from build123d import *

# Parameters (mm, degrees)
EXTRUDE_1_DEPTH     = 6
EXTRUDE_2_DEPTH     = 20
SKETCH_3_W          = 25
SKETCH_3_H          = 50
EXTRUDE_3_DEPTH     = 3
EXTRUDE_4_DEPTH     = 6
SKETCH_5_R          = 1
CUT_EXTRUDE_1_DEPTH = 74.184697854


with BuildPart() as part:
    # 草图1 → 凸台-拉伸1 (new body)
    with BuildSketch(Plane(origin=(0, 0, 0), x_dir=(1, 0, 0), z_dir=(0, 1, 0))):
        with BuildLine():
            Line((5, 0), (5, -13))
            Line((5, -13), (-15, -13))
            Line((-15, -13), (-15, -63))
            Line((-15, -63), (10, -63))
            Line((10, -63), (10, -66))
            Line((10, -66), (-18, -66))
            Line((-18, -66), (-18, -10))
            Line((-18, -10), (-5, -10))
            Line((-5, -10), (-5, 0))
            ThreePointArc((-5, 0), (0, 5), (5, 0))
        make_face()
    extrude(amount=-EXTRUDE_1_DEPTH)

    # 草图2 → 凸台-拉伸2 (add, symmetric)
    with BuildSketch(Plane(origin=(0, 0, 0), x_dir=(1, 0, 0), z_dir=(0, 1, 0))):
        Polygon((-15, -13), (5, -13), (5, -10), (-18, -10), (-18, -66), (10, -66), (10, -63), (-15, -63), align=None)
    extrude(amount=EXTRUDE_2_DEPTH, both=True)

    # 草图3 → 凸台-拉伸3 (add)
    with BuildSketch(Plane.XZ.offset(20)):
        with Locations((-2.5, 38)):
            Rectangle(SKETCH_3_W, SKETCH_3_H)
    extrude(amount=-EXTRUDE_3_DEPTH)

    # 草图4 → 凸台-拉伸4 (add)
    with BuildSketch(Plane.XZ.offset(6)):
        with BuildLine():
            ThreePointArc((0.860680542, 8.706562468), (0.72579344, 9.898750182), (0.24342364, 10.997306258))
            ThreePointArc((0.24342364, 10.997306258), (-0.01511058, 10.999989621), (-0.273636452, 10.996595977))
            ThreePointArc((-0.273636452, 10.996595977), (-0.752986286, 9.896718796), (-0.884597491, 8.704164996))
            ThreePointArc((-0.884597491, 8.704164996), (-1.380514283, 8.639397046), (-1.871919927, 8.546397884))
            ThreePointArc((-1.871919927, 8.546397884), (-2.368611449, 9.638553371), (-3.166844887, 10.53428182))
            ThreePointArc((-3.166844887, 10.53428182), (-3.413554747, 10.456942383), (-3.658378768, 10.373825947))
            ThreePointArc((-3.658378768, 10.373825947), (-3.77438681, 9.179653342), (-3.531037114, 8.00479718))
            ThreePointArc((-3.531037114, 8.00479718), (-3.982667613, 7.789952483), (-4.421283831, 7.549652329))
            ThreePointArc((-4.421283831, 7.549652329), (-5.231160146, 8.434867801), (-6.267120572, 9.040088481))
            ThreePointArc((-6.267120572, 9.040088481), (-6.477856391, 8.890296766), (-6.685013481, 8.735593555))
            ThreePointArc((-6.685013481, 8.735593555), (-6.426324056, 7.564019461), (-5.831834222, 6.521864044))
            ThreePointArc((-5.831834222, 6.521864044), (-6.194969688, 6.177973095), (-6.537861669, 5.813894202))
            ThreePointArc((-6.537861669, 5.813894202), (-7.58164644, 6.405518601), (-8.753926829, 6.660988295))
            ThreePointArc((-8.753926829, 6.660988295), (-8.908060318, 6.453406959), (-9.057272497, 6.242260401))
            ThreePointArc((-9.057272497, 6.242260401), (-8.449207929, 5.207966653), (-7.561770763, 4.400525414))
            ThreePointArc((-7.561770763, 4.400525414), (-7.800864967, 3.961250657), (-8.014468055, 3.509031603))
            ThreePointArc((-8.014468055, 3.509031603), (-9.189988356, 3.74915261), (-10.383837737, 3.629864165))
            ThreePointArc((-10.383837737, 3.629864165), (-10.466281235, 3.384812715), (-10.542942575, 3.137891306))
            ThreePointArc((-10.542942575, 3.137891306), (-9.64502446, 2.342121783), (-8.551508496, 1.848432697))
            ThreePointArc((-8.551508496, 1.848432697), (-8.643157232, 1.356773404), (-8.706562468, 0.860680542))
            ThreePointArc((-8.706562468, 0.860680542), (-9.898750182, 0.72579344), (-10.997306258, 0.24342364))
            ThreePointArc((-10.997306258, 0.24342364), (-10.999989621, -0.01511058), (-10.996595977, -0.273636452))
            ThreePointArc((-10.996595977, -0.273636452), (-9.896718796, -0.752986286), (-8.704164996, -0.884597491))
            ThreePointArc((-8.704164996, -0.884597491), (-8.639397046, -1.380514283), (-8.546397884, -1.871919927))
            ThreePointArc((-8.546397884, -1.871919927), (-9.638553371, -2.368611449), (-10.53428182, -3.166844887))
            ThreePointArc((-10.53428182, -3.166844887), (-10.456942383, -3.413554747), (-10.373825947, -3.658378768))
            ThreePointArc((-10.373825947, -3.658378768), (-9.179653342, -3.77438681), (-8.00479718, -3.531037114))
            ThreePointArc((-8.00479718, -3.531037114), (-7.789952483, -3.982667613), (-7.549652329, -4.421283831))
            ThreePointArc((-7.549652329, -4.421283831), (-8.434867801, -5.231160146), (-9.040088481, -6.267120572))
            ThreePointArc((-9.040088481, -6.267120572), (-8.890296766, -6.477856391), (-8.735593555, -6.685013481))
            ThreePointArc((-8.735593555, -6.685013481), (-7.564019461, -6.426324056), (-6.521864044, -5.831834222))
            ThreePointArc((-6.521864044, -5.831834222), (-6.177973095, -6.194969688), (-5.813894202, -6.537861669))
            ThreePointArc((-5.813894202, -6.537861669), (-6.405518601, -7.58164644), (-6.660988295, -8.753926829))
            ThreePointArc((-6.660988295, -8.753926829), (-6.453406959, -8.908060318), (-6.242260401, -9.057272497))
            ThreePointArc((-6.242260401, -9.057272497), (-5.207966653, -8.449207929), (-4.400525414, -7.561770763))
            ThreePointArc((-4.400525414, -7.561770763), (-3.961250657, -7.800864967), (-3.509031603, -8.014468055))
            ThreePointArc((-3.509031603, -8.014468055), (-3.74915261, -9.189988356), (-3.629864165, -10.383837737))
            ThreePointArc((-3.629864165, -10.383837737), (-3.384812715, -10.466281235), (-3.137891306, -10.542942575))
            ThreePointArc((-3.137891306, -10.542942575), (-2.342121783, -9.64502446), (-1.848432697, -8.551508496))
            ThreePointArc((-1.848432697, -8.551508496), (-1.356773404, -8.643157232), (-0.860680542, -8.706562468))
            ThreePointArc((-0.860680542, -8.706562468), (-0.72579344, -9.898750182), (-0.24342364, -10.997306258))
            ThreePointArc((-0.24342364, -10.997306258), (0.01511058, -10.999989621), (0.273636452, -10.996595977))
            ThreePointArc((0.273636452, -10.996595977), (0.752986286, -9.896718796), (0.884597491, -8.704164996))
            ThreePointArc((0.884597491, -8.704164996), (1.380514283, -8.639397046), (1.871919927, -8.546397884))
            ThreePointArc((1.871919927, -8.546397884), (2.368611449, -9.638553371), (3.166844887, -10.53428182))
            ThreePointArc((3.166844887, -10.53428182), (3.413554747, -10.456942383), (3.658378768, -10.373825947))
            ThreePointArc((3.658378768, -10.373825947), (3.77438681, -9.179653342), (3.531037114, -8.00479718))
            ThreePointArc((3.531037114, -8.00479718), (3.982667613, -7.789952483), (4.421283831, -7.549652329))
            ThreePointArc((4.421283831, -7.549652329), (5.231160146, -8.434867801), (6.267120572, -9.040088481))
            ThreePointArc((6.267120572, -9.040088481), (6.477856391, -8.890296766), (6.685013481, -8.735593555))
            ThreePointArc((6.685013481, -8.735593555), (6.426324056, -7.564019461), (5.831834222, -6.521864044))
            ThreePointArc((5.831834222, -6.521864044), (6.194969688, -6.177973095), (6.537861669, -5.813894202))
            ThreePointArc((6.537861669, -5.813894202), (7.58164644, -6.405518601), (8.753926829, -6.660988295))
            ThreePointArc((8.753926829, -6.660988295), (8.908060318, -6.453406959), (9.057272497, -6.242260401))
            ThreePointArc((9.057272497, -6.242260401), (8.449207929, -5.207966653), (7.561770763, -4.400525414))
            ThreePointArc((7.561770763, -4.400525414), (7.800864967, -3.961250657), (8.014468055, -3.509031603))
            ThreePointArc((8.014468055, -3.509031603), (9.189988356, -3.74915261), (10.383837737, -3.629864165))
            ThreePointArc((10.383837737, -3.629864165), (10.466281235, -3.384812715), (10.542942575, -3.137891306))
            ThreePointArc((10.542942575, -3.137891306), (9.64502446, -2.342121783), (8.551508496, -1.848432697))
            ThreePointArc((8.551508496, -1.848432697), (8.643157232, -1.356773404), (8.706562468, -0.860680542))
            ThreePointArc((8.706562468, -0.860680542), (9.898750182, -0.72579344), (10.997306258, -0.24342364))
            ThreePointArc((10.997306258, -0.24342364), (10.999989621, 0.01511058), (10.996595977, 0.273636452))
            ThreePointArc((10.996595977, 0.273636452), (9.896718796, 0.752986286), (8.704164996, 0.884597491))
            ThreePointArc((8.704164996, 0.884597491), (8.639397046, 1.380514283), (8.546397884, 1.871919927))
            ThreePointArc((8.546397884, 1.871919927), (9.638553371, 2.368611449), (10.53428182, 3.166844887))
            ThreePointArc((10.53428182, 3.166844887), (10.456942383, 3.413554747), (10.373825947, 3.658378768))
            ThreePointArc((10.373825947, 3.658378768), (9.179653342, 3.77438681), (8.00479718, 3.531037114))
            ThreePointArc((8.00479718, 3.531037114), (7.789952483, 3.982667613), (7.549652329, 4.421283831))
            ThreePointArc((7.549652329, 4.421283831), (8.434867801, 5.231160146), (9.040088481, 6.267120572))
            ThreePointArc((9.040088481, 6.267120572), (8.890296766, 6.477856391), (8.735593555, 6.685013481))
            ThreePointArc((8.735593555, 6.685013481), (7.564019461, 6.426324056), (6.521864044, 5.831834222))
            ThreePointArc((6.521864044, 5.831834222), (6.177973095, 6.194969688), (5.813894202, 6.537861669))
            ThreePointArc((5.813894202, 6.537861669), (6.405518601, 7.58164644), (6.660988295, 8.753926829))
            ThreePointArc((6.660988295, 8.753926829), (6.453406959, 8.908060318), (6.242260401, 9.057272497))
            ThreePointArc((6.242260401, 9.057272497), (5.207966653, 8.449207929), (4.400525414, 7.561770763))
            ThreePointArc((4.400525414, 7.561770763), (3.961250657, 7.800864967), (3.509031603, 8.014468055))
            ThreePointArc((3.509031603, 8.014468055), (3.74915261, 9.189988356), (3.629864165, 10.383837737))
            ThreePointArc((3.629864165, 10.383837737), (3.384812715, 10.466281235), (3.137891306, 10.542942575))
            ThreePointArc((3.137891306, 10.542942575), (2.342121783, 9.64502446), (1.848432697, 8.551508496))
            ThreePointArc((1.848432697, 8.551508496), (1.356773404, 8.643157232), (0.860680542, 8.706562468))
        make_face()
    extrude(amount=-EXTRUDE_4_DEPTH)

    # 草图5 → 切除-拉伸1 (cut, through all)
    with BuildSketch(Plane.XZ.offset(6)):
        with Locations(Location((0, 6.5, 0), (0, 0, 270))):
            Circle(SKETCH_5_R)
        with Locations(Location((0, -6.5, 0), (0, 0, 270))):
            Circle(SKETCH_5_R)
    extrude(amount=-CUT_EXTRUDE_1_DEPTH, mode=Mode.SUBTRACT)


solid = part.part
Can you work these out from the model? Positions are in its coordinate system, mm. A direction names the side the tool comes from. Coordinates: 2 decimals unless noted, no trailing zeros. Write each loop counter-clockwise with the first axis right and the second up, starting at its lowest first coordinate (ties: lowest second). Pieces come first, ordered by that corner, then holes. Notation, with made-up numbers: (12.25, -36) -> (26.25, -36) arc R20 cw to (26.25, -19) -> close; hole circle Ø3 at (89, -15.5). An arc over 180 degrees is marked (long way). Write each question's results on one line, items separated by ' | '. Start each with the question number.
Q1. Imagine slicing it at B-B (y = 5). Write out the boundary of the cut face in (x, z), then the cut area to 3 significant figures.
Q2. If I drill on probe 1 along Z at (x, y) = (-1.5, -7.5); probe 2 along Y at (x, z) = (6.5, 48.5); probe 3 along X at (y, z) = (-1, 6) (1 decimal), over which ranges is the centre line in solid material (lowest first)?
Q3. Imagine slicing it at A-A (x = -14.25). Write out the boundary of the cut face in (y, z), then the cut area to 3 significant figures.
Q4. Imagine slicing it at C-C (z = 38.5). Write out the boundary of the cut face in (x, y).
Q5. On a 3-axis mill with a long thin cutter (end or side, diameter ignored), from which of +Z, -Z, +X, -X, +Y, -Y can I reach the whole of each face in a straight line? I mean faces 5 (the face through (5.218, -3.042, -8.424)), 6 (the face through (-3, -17, 38)), 7 (the face through (-8.424, -3.042, -5.218)). Say none if no direction works.
Q6. I'm going to push flat-ended pins straight in: pin 1 (7 mm diameter, centred on x = -11, y = -5, fed in from -Z) (3 decimals); pin 2 (0.5 mm diameter, centred on y = -3, z = 8.5, fed in from -X) (3 decimals); pin 3 (12.5 mm diameter, centred on x = 0, z = 44, fed in from +Y). Where does each tip first touch, or does it pass through?
Q7. We'd pull the mould along X, two halves only. Please class faces 1 (the face through (8.46, -3.04, -5.22)), 2 (the face through (-8.46, -3.04, 5.22)), 3 (the face through (-7.58, -3.042, -6.432)), 4 (the face through (-6, 0, 10)): +X half, -X half, draft (parallel to the pull), parting line (faces both ways), or undercut.
Taken from the geometry:
1) outline: (-18, 10) -> (5, 10) -> (5, 13) -> (-15, 13) -> (-15, 63) -> (10, 63) -> (10, 66) -> (-18, 66) -> close | area: 303 mm^2
2) probe 1: z = 10 to 13, 63 to 66 | probe 2: y = -20 to -17 | probe 3: x = -9 to -6.8, -6.4 to -0.9, 0.9 to 6.4, 6.8 to 8.9
3) outline: (-20, 10) -> (20, 10) -> (20, 13) -> (-17, 13) -> (-17, 63) -> (20, 63) -> (20, 66) -> (-20, 66) -> close | area: 390 mm^2
4) outline: (-18, -20) -> (10, -20) -> (10, -17) -> (-15, -17) -> (-15, 20) -> (-18, 20) -> close
5) face 5: -Z, +Y, -Y | face 6: +X, +Y | face 7: -X, +Y, -Y
6) pin 1: stops at z = -6.685 | pin 2: stops at x = -6.685 | pin 3: stops at y = -17
7) face 1: +X half | face 2: -X half | face 3: undercut | face 4: draft
